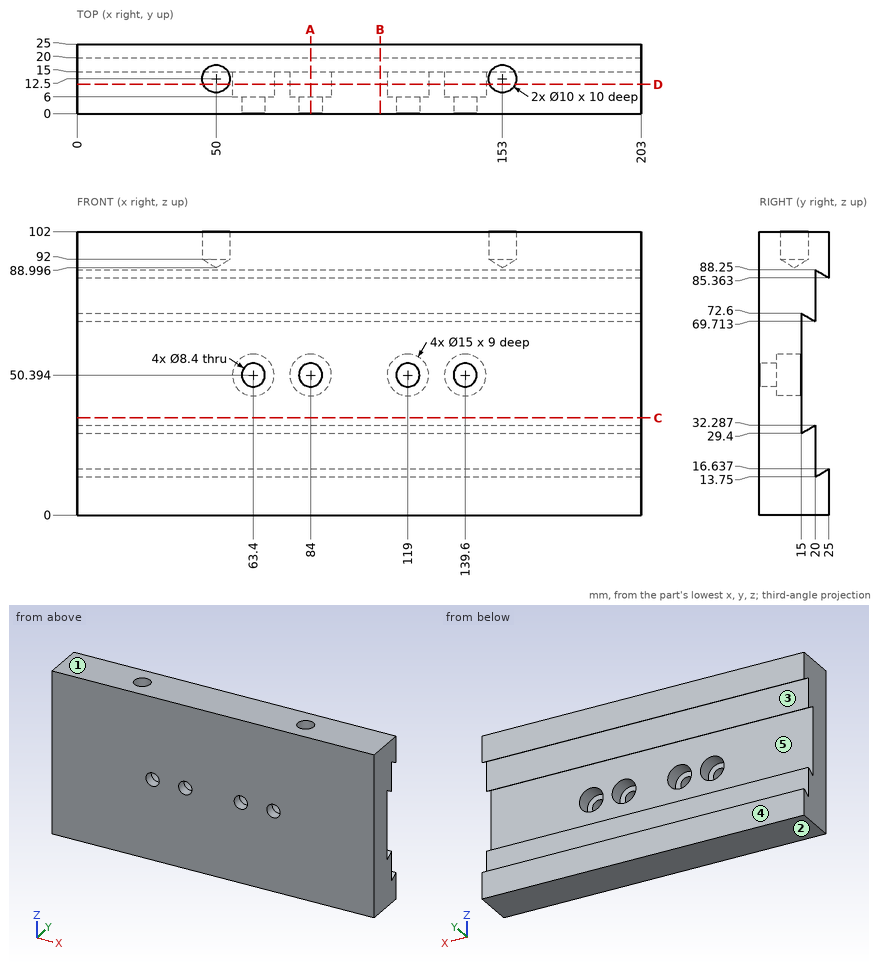
Design review of the part shown in the three views and the two pictorial views. Dimensions are in mm from the part's minimum x, y and z. A direction names the side the tool comes from. Round coordinates to 2 decimals unless told otherwise and drop trailing zeros. Write each loop counter-clockwise with the first axis right and the second up, starting at its lowest first coordinate (ties: lowest second). Pieces come first, ordered by that corner, then holes. Notation, with made-up numbers: (3, -1.75) -> (7, -1.75) arc R17 ccw to (7, 24.25) -> close; hole circle Ø8 at (89.5, 43). An arc over 180 degrees is marked (long way). One line per question, with ' | ' between items. Start each with the question number.
1) Add section A-A (x = 84). Write out the cut boundary in (y, z), and give its area (4 significant figures).
2) Mouldability with a two-part tool opening along Z and no side actions: class the marked faces 1, 2 and 3 as +Z half, -Z half, draft (parallel to the pull), parting line (faces both ways), or undercut.
3) Wall thickness on line 1 along X through (y, z) = (12.5, 97.25); line 2 along Z through (x, y) = (84, 12); line 3 along Y through (x, z) = (182, 36): over which ranges is each line inside the solid? List them lowest first.
4) Machinability: for the marked faces 4 and 5, which of the approach directions +Z, -Z, +X, -X, +Y, -Y give a long, thin tool a straight path to every point of the face, cutting with its end or side? Answer none if there is none.
5) Add section D-D (y = 10.5). Count the separate pieces of the cut face and the enclosed holes in it, and give its area (3 significant figures).
6) Add section B-B (x = 109). Write out the cut boundary in (y, z), and give its area (3 significant figures).
7) For pin 1 Ø12 at (x, z) = (84, 50.39) entering from -Y; pin 2 Ø16.5 at (x, z) = (121.5, 52) entering from +Y; pin 3 Ø4.5 at (x, z) = (63.5, 50) entering from +Y; pin 4 Ø11 at (x, z) = (139.6, 50.39) entering from +Y, all flat-tipped, find the tip position at first contact; note any pin that passes through.
8) Add section C-C (z = 35). Write out the cut boundary in (x, y).
Reported:
1) outline: (0, 0) -> (25, 0) -> (25, 16.64) -> (20, 13.75) -> (20, 32.29) -> (15, 29.4) -> (15, 42.89) -> (6, 42.89) -> (6, 46.19) -> (0, 46.19) -> close; (0, 54.59) -> (6, 54.59) -> (6, 57.89) -> (15, 57.89) -> (15, 72.6) -> (20, 69.71) -> (20, 88.25) -> (25, 85.36) -> (25, 102) -> (0, 102) -> close | area: 1,805 mm²
2) face 1: +Z half | face 2: -Z half | face 3: undercut
3) line 1: x = 0 to 45, 55 to 148, 158 to 203 | line 2: z = 0 to 42.89, 57.89 to 102 | line 3: y = 0 to 15
4) face 4: +Z, -Z, +X, -X, +Y | face 5: +X, -X
5) separate pieces: 1 | enclosed holes: 4 | area: 19,800 mm²
6) outline: (0, 0) -> (25, 0) -> (25, 16.64) -> (20, 13.75) -> (20, 32.29) -> (15, 29.4) -> (15, 72.6) -> (20, 69.71) -> (20, 88.25) -> (25, 85.36) -> (25, 102) -> (0, 102) -> close | area: 1,990 mm²
7) pin 1: stops at y = 0 | pin 2: stops at y = 15 | pin 3: passes through | pin 4: stops at y = 6
8) outline: (0, 0) -> (203, 0) -> (203, 15) -> (0, 15) -> close
